The model under review builds one solid part; all positions refer to its coordinate system, in mm. A direction names the side the tool comes from. Coordinates: 2 decimals unless noted, no trailing zeros. Write each loop counter-clockwise with the first axis right and the second up, starting at its lowest first coordinate (ties: lowest second). Pieces come first, ordered by that corner, then holes.
1) Mouldability with a two-part tool opening along Y and no side actions: class faces 1 (the cylindrical face through (4.67, -0.76, 101.48)), 2 (the flat face through (14.42, 4.31, 52.75)), 3 (the cylindrical face through (18.3, 17.6, 15.5)) as released by +Y, released by -Y, zero draft, split by the parting line, or undercut.
2) Add section D-D, the plane z = 20. State the section outline as (x, y) points.
3) For line 1 (Z direction, x = 5, y = 35.7); line 2 (Y direction, x = 6.5, z = 70); line 3 (Y direction, x = 17, z = 47.5), list the stretches that pass through material, from the lowest coordinate up.
4) Add section B-B, the plane x = 5. State the section outline as (y, z) points.
5) Machinability: for faces 4 (the cylindrical face through (18.26, 18.701, 66.185)), 5 (the flat face through (4, 0, 53)), which of the approach directions +Z, -Z, +X, -X, +Y, -Y give a long, thin tool a straight path to every point of the face, cutting with its end or side? Answer none if there is none.
6) For P1, Ø5, axis at x = 11, z = 26, coming from the -Y side; P2, Ø9.5, axis at y = 17.5, z = 40, coming from the -X side; P3, Ø2, axis at y = 5, z = 12.5, coming from the -X side; P4, Ø8, axis at x = 16.5, z = 28, coming from the +Y side, all flat-tipped, find the tip position at first contact; note any pin that passes through.
7) Add section C-C, the plane z = 99. State the section outline as (x, y) points, then the cut area to 3 significant figures.
8) Add section A-A, the plane z = 40. State the section outline as (x, y) points.
from build123d import *

# Parameters (mm, degrees)
SALIENTE_EXTRUIR1_DEPTH = 107
CORTAR_EXTRUIR1_REACH   = 40
CROQUIS3_R              = 2.5
CORTAR_EXTRUIR2_REACH   = 40
CROQUIS4_R              = 2.5
CORTAR_EXTRUIR3_REACH   = 21
CROQUIS5_R              = 3
CROQUIS5_R_2            = 4
CORTAR_EXTRUIR4_REACH   = 21
CROQUIS6_R              = 6.5
CORTAR_EXTRUIR5_REACH   = 21
CROQUIS7_R              = 2.5


with BuildPart() as part:
    # Croquis1 → Saliente-Extruir1 (new body)
    with BuildSketch(Plane.XY):
        Polygon((0, 0), (9, 0), (17.5, 10.5), (17.5, 24.5), (9, 35), (0, 35), (0, 36.5), (9.715608012, 36.5), (19, 25.031045192), (19, 9.968954808), (9.715608012, -1.5), (0, -1.5), align=None)
    extrude(amount=SALIENTE_EXTRUIR1_DEPTH)

    # Croquis3 → Cortar-Extruir1 (cut, up to next)
    with BuildSketch(Plane(origin=(0, 36.5, 0), x_dir=(1, 0, 0), z_dir=(0, 1, 0)), mode=Mode.PRIVATE) as cortar_extruir1_sk1:
        with Locations((5, -8)):
            Circle(CROQUIS3_R)
    cortar_extruir1_tool1 = extrude(cortar_extruir1_sk1.sketch, amount=-CORTAR_EXTRUIR1_REACH, mode=Mode.PRIVATE) & part.part
    add(cortar_extruir1_tool1.solids().sort_by_distance((5, 36.5, 8))[0], mode=Mode.SUBTRACT)
    # Croquis3 → Cortar-Extruir1 (cut, up to next)
    with BuildSketch(Plane(origin=(0, 36.5, 0), x_dir=(1, 0, 0), z_dir=(0, 1, 0)), mode=Mode.PRIVATE) as cortar_extruir1_sk2:
        with Locations((5, -99)):
            Circle(CROQUIS3_R)
    cortar_extruir1_tool2 = extrude(cortar_extruir1_sk2.sketch, amount=-CORTAR_EXTRUIR1_REACH, mode=Mode.PRIVATE) & part.part
    add(cortar_extruir1_tool2.solids().sort_by_distance((5, 36.5, 99))[0], mode=Mode.SUBTRACT)

    # Croquis4 → Cortar-Extruir2 (cut, up to next)
    with BuildSketch(Plane.XZ.offset(1.5), mode=Mode.PRIVATE) as cortar_extruir2_sk1:
        with Locations((5, 8)):
            Circle(CROQUIS4_R)
    cortar_extruir2_tool1 = extrude(cortar_extruir2_sk1.sketch, amount=-CORTAR_EXTRUIR2_REACH, mode=Mode.PRIVATE) & part.part
    add(cortar_extruir2_tool1.solids().sort_by_distance((5, -1.5, 8))[0], mode=Mode.SUBTRACT)
    # Croquis4 → Cortar-Extruir2 (cut, up to next)
    with BuildSketch(Plane.XZ.offset(1.5), mode=Mode.PRIVATE) as cortar_extruir2_sk2:
        with Locations((5, 99)):
            Circle(CROQUIS4_R)
    cortar_extruir2_tool2 = extrude(cortar_extruir2_sk2.sketch, amount=-CORTAR_EXTRUIR2_REACH, mode=Mode.PRIVATE) & part.part
    add(cortar_extruir2_tool2.solids().sort_by_distance((5, -1.5, 99))[0], mode=Mode.SUBTRACT)

    # Croquis5 → Cortar-Extruir3 (cut, up to next)
    with BuildSketch(Plane(origin=(19, 0, 0), x_dir=(0, 0, -1), z_dir=(1, 0, 0)), mode=Mode.PRIVATE) as cortar_extruir3_sk1:
        with Locations((-40, 17.5)):
            Circle(CROQUIS5_R)
    cortar_extruir3_tool1 = extrude(cortar_extruir3_sk1.sketch, amount=-CORTAR_EXTRUIR3_REACH, mode=Mode.PRIVATE) & part.part
    add(cortar_extruir3_tool1.solids().sort_by_distance((19, 17.5, 40))[0], mode=Mode.SUBTRACT)
    # Croquis5 → Cortar-Extruir3 (cut, up to next)
    with BuildSketch(Plane(origin=(19, 0, 0), x_dir=(0, 0, -1), z_dir=(1, 0, 0)), mode=Mode.PRIVATE) as cortar_extruir3_sk2:
        with Locations((-70, 17.5)):
            Circle(CROQUIS5_R_2)
    cortar_extruir3_tool2 = extrude(cortar_extruir3_sk2.sketch, amount=-CORTAR_EXTRUIR3_REACH, mode=Mode.PRIVATE) & part.part
    add(cortar_extruir3_tool2.solids().sort_by_distance((19, 17.5, 70))[0], mode=Mode.SUBTRACT)

    # Croquis6 → Cortar-Extruir4 (cut, up to next)
    with BuildSketch(Plane(origin=(19, 0, 0), x_dir=(0, 0, -1), z_dir=(1, 0, 0)), mode=Mode.PRIVATE) as cortar_extruir4_sk1:
        with Locations((-52.395650843, 17.501045192)):
            Circle(CROQUIS6_R)
    cortar_extruir4_tool1 = extrude(cortar_extruir4_sk1.sketch, amount=-CORTAR_EXTRUIR4_REACH, mode=Mode.PRIVATE) & part.part
    add(cortar_extruir4_tool1.solids().sort_by_distance((19, 17.501045, 52.395651))[0], mode=Mode.SUBTRACT)

    # Croquis7 → Cortar-Extruir5 (cut, up to next)
    with BuildSketch(Plane(origin=(19, 0, 0), x_dir=(0, 0, -1), z_dir=(1, 0, 0)), mode=Mode.PRIVATE) as cortar_extruir5_sk1:
        with Locations((-27, 17.503954808)):
            Circle(CROQUIS7_R)
    cortar_extruir5_tool1 = extrude(cortar_extruir5_sk1.sketch, amount=-CORTAR_EXTRUIR5_REACH, mode=Mode.PRIVATE) & part.part
    add(cortar_extruir5_tool1.solids().sort_by_distance((19, 17.503955, 27))[0], mode=Mode.SUBTRACT)
    # Croquis7 → Cortar-Extruir5 (cut, up to next)
    with BuildSketch(Plane(origin=(19, 0, 0), x_dir=(0, 0, -1), z_dir=(1, 0, 0)), mode=Mode.PRIVATE) as cortar_extruir5_sk2:
        with Locations((-20, 17.503954808)):
            Circle(CROQUIS7_R)
    cortar_extruir5_tool2 = extrude(cortar_extruir5_sk2.sketch, amount=-CORTAR_EXTRUIR5_REACH, mode=Mode.PRIVATE) & part.part
    add(cortar_extruir5_tool2.solids().sort_by_distance((19, 17.503955, 20))[0], mode=Mode.SUBTRACT)
    # Croquis7 → Cortar-Extruir5 (cut, up to next)
    with BuildSketch(Plane(origin=(19, 0, 0), x_dir=(0, 0, -1), z_dir=(1, 0, 0)), mode=Mode.PRIVATE) as cortar_extruir5_sk3:
        with Locations((-13, 17.503954808)):
            Circle(CROQUIS7_R)
    cortar_extruir5_tool3 = extrude(cortar_extruir5_sk3.sketch, amount=-CORTAR_EXTRUIR5_REACH, mode=Mode.PRIVATE) & part.part
    add(cortar_extruir5_tool3.solids().sort_by_distance((19, 17.503955, 13))[0], mode=Mode.SUBTRACT)


solid = part.part
Geometry results:
1. face 1: zero draft
1. face 2: released by -Y
1. face 3: undercut
2. outline: (0, -1.5) - (9.72, -1.5) - (19, 9.97) - (19, 15) - (17.5, 15) - (17.5, 10.5) - (9, 0) - (0, 0) - close; (0, 35) - (9, 35) - (17.5, 24.5) - (17.5, 20) - (19, 20) - (19, 25.03) - (9.72, 36.5) - (0, 36.5) - close
3. line 1: z = 0 to 5.5, 10.5 to 96.5, 101.5 to 107
3. line 2: y = -1.5 to 0, 35 to 36.5
3. line 3: y = 7.5 to 9.88, 25.12 to 27.5
4. outline: (-1.5, 0) - (0, 0) - (0, 5.5) - (-1.5, 5.5) - close; (-1.5, 10.5) - (0, 10.5) - (0, 96.5) - (-1.5, 96.5) - close; (-1.5, 101.5) - (0, 101.5) - (0, 107) - (-1.5, 107) - close; (35, 0) - (36.5, 0) - (36.5, 5.5) - (35, 5.5) - close; (35, 10.5) - (36.5, 10.5) - (36.5, 96.5) - (35, 96.5) - close; (35, 101.5) - (36.5, 101.5) - (36.5, 107) - (35, 107) - close
5. face 4: +X, -X
5. face 5: +Z, -Z, -X
6. P1: stops at y = -1.5
6. P2: stops at x = 17.5
6. P3: stops at x = 12.24
6. P4: stops at y = 33.06
7. outline: (0, -1.5) - (2.5, -1.5) - (2.5, 0) - (0, 0) - close; (0, 35) - (2.5, 35) - (2.5, 36.5) - (0, 36.5) - close; (7.5, -1.5) - (9.72, -1.5) - (19, 9.97) - (19, 25.03) - (9.72, 36.5) - (7.5, 36.5) - (7.5, 35) - (9, 35) - (17.5, 24.5) - (17.5, 10.5) - (9, 0) - (7.5, 0) - close
7. area: 77.3 mm2
8. outline: (0, -1.5) - (9.72, -1.5) - (19, 9.97) - (19, 14.5) - (17.5, 14.5) - (17.5, 10.5) - (9, 0) - (0, 0) - close; (0, 35) - (9, 35) - (17.5, 24.5) - (17.5, 20.5) - (19, 20.5) - (19, 25.03) - (9.72, 36.5) - (0, 36.5) - close
